```python
from build123d import *

# Parameters (mm, degrees)
ESBO_O1_W                = 35
ESBO_O1_H                = 20
RESSALTO_EXTRUS_O1_DEPTH = 5
ESBO_O2_W                = 5
ESBO_O2_H                = 20
RESSALTO_EXTRUS_O2_DEPTH = 30
ESBO_O4_W                = 42.3
ESBO_O4_H                = 5
RESSALTO_EXTRUS_O3_DEPTH = 50
ESBO_O5_W                = 7.3
ESBO_O5_H                = 5
RESSALTO_EXTRUS_O4_DEPTH = 35
ESBO_O6_R                = 3.1
ESBO_O6_R_2              = 12.5
CORTE_EXTRUS_O1_DEPTH    = 39
ESBO_O7_R                = 3
CORTE_EXTRUS_O2_DEPTH    = 36
ESBO_O8_R                = 3
CORTE_EXTRUS_O3_DEPTH    = 10


with BuildPart() as part:
    # Esboço1 → Ressalto-extrusão1 (new body)
    with BuildSketch(Plane.XY):
        with Locations((-76.705213928, -265)):
            Rectangle(ESBO_O1_W, ESBO_O1_H)
    extrude(amount=RESSALTO_EXTRUS_O1_DEPTH)

    # Esboço2 → Ressalto-extrusão2 (add)
    with BuildSketch(Plane(origin=(0, 0, 0), x_dir=(-1, 0, 0), z_dir=(0, 0, -1))):
        with Locations((61.705213928, -265)):
            Rectangle(ESBO_O2_W, ESBO_O2_H)
    extrude(amount=RESSALTO_EXTRUS_O2_DEPTH)

    # Esboço4 → Ressalto-extrusão3 (add)
    with BuildSketch(Plane(origin=(-59.205213928, 0, 0), x_dir=(0, 0, -1), z_dir=(1, 0, 0))):
        with Locations((8.85, -272.5)):
            Rectangle(ESBO_O4_W, ESBO_O4_H)
    extrude(amount=RESSALTO_EXTRUS_O3_DEPTH)

    # Esboço5 → Ressalto-extrusão4 (add)
    with BuildSketch(Plane.ZY.offset(59.205213928)):
        with Locations((8.65, -272.5)):
            Rectangle(ESBO_O5_W, ESBO_O5_H)
    extrude(amount=RESSALTO_EXTRUS_O4_DEPTH)

    # Esboço6 → Corte-extrusão1 (cut)
    with BuildSketch(Plane.XZ.offset(275)):
        with Locations((-14.555213928, 6.65)):
            Circle(ESBO_O6_R)
        with Locations((-45.555213928, -24.35)):
            Circle(ESBO_O6_R)
        with Locations((-30.055213928, -8.85)):
            Circle(ESBO_O6_R_2)
        with Locations((-45.555213928, 6.65)):
            Circle(ESBO_O6_R)
        with Locations((-14.555213928, -24.35)):
            Circle(ESBO_O6_R)
    extrude(amount=-CORTE_EXTRUS_O1_DEPTH, mode=Mode.SUBTRACT)

    # Esboço7 → Corte-extrusão2 (cut, through all)
    with BuildSketch(Plane(origin=(-59.205213928, 0, 0), x_dir=(0, 0, -1), z_dir=(1, 0, 0))):
        with Locations((21, -262.5)):
            Circle(ESBO_O7_R)
        with Locations((7, -262.5)):
            Circle(ESBO_O7_R)
    extrude(amount=-CORTE_EXTRUS_O2_DEPTH, mode=Mode.SUBTRACT)

    # Esboço8 → Corte-extrusão3 (cut)
    with BuildSketch(Plane.XY.offset(5)):
        with Locations((-71.205213928, -262.5)):
            Circle(ESBO_O8_R)
        with Locations((-86.205213928, -262.5)):
            Circle(ESBO_O8_R)
    extrude(amount=-CORTE_EXTRUS_O3_DEPTH, mode=Mode.SUBTRACT)


solid = part.part
```
Can you work these out from the model? Positions are in its coordinate system, mm. A direction names the side the tool comes from. Coordinates: 2 decimals unless noted, no trailing zeros. Loops run counter-clockwise (first coordinate to the right, second up) from the corner with the lowest first, then second, coordinate; pieces in that order, holes last. Notation, with made-up numbers: (43, 6) - (48, 6) arc R14 ccw to (48, 24) - close; hole circle Ø8 at (84, 70.5). An arc over 180 degrees is marked (long way). Use a Markdown table: item, result.
Item 1: I want a section at C-C on z = -2.5. Please give me the cut outline in (x, y).
Numbers:
| item | result |
|---|---|
| outline | (-64.21, -275) - (-40.82, -275) - (-40.82, -270) - (-59.21, -270) - (-59.21, -255) - (-64.21, -255) - close; (-19.29, -275) - (-9.21, -275) - (-9.21, -270) - (-19.29, -270) - close |
Item 2: I want a section at D-D on x = -85.5. Please give me the cut outline in (y, z), and give its area (3 significant figures).
Numbers:
| item | result |
|---|---|
| outline | (-275, 0) - (-265.42, 0) - (-265.42, 5) - (-270, 5) - (-270, 12.3) - (-275, 12.3) - close; (-259.58, 0) - (-255, 0) - (-255, 5) - (-259.58, 5) - close |
| area | 107 mm2 |
Item 3: I want a section at A-A on y = -262.5. Please give me the cut outline in (x, z).
Numbers:
| item | result |
|---|---|
| outline | (-94.21, 0) - (-89.21, 0) - (-89.21, 5) - (-94.21, 5) - close; (-83.21, 0) - (-74.21, 0) - (-74.21, 5) - (-83.21, 5) - close; (-68.21, 0) - (-64.21, 0) - (-64.21, -4) - (-59.21, -4) - (-59.21, 5) - (-68.21, 5) - close; (-64.21, -30) - (-59.21, -30) - (-59.21, -24) - (-64.21, -24) - close; (-64.21, -18) - (-59.21, -18) - (-59.21, -10) - (-64.21, -10) - close |
Item 4: I want a section at B-B on z = -8.85. Please give me the cut outline in (x, y), and give its area (3 significant figures).
Numbers:
| item | result |
|---|---|
| outline | (-64.21, -275) - (-42.56, -275) - (-42.56, -270) - (-59.21, -270) - (-59.21, -264.86) - (-64.21, -264.86) - close; (-64.21, -260.14) - (-59.21, -260.14) - (-59.21, -255) - (-64.21, -255) - close; (-17.56, -275) - (-9.21, -275) - (-9.21, -270) - (-17.56, -270) - close |
| area | 201 mm2 |
Item 5: For faces 5 (the face through (-18.13, -272.54, -5.1)), 6 (the face through (-79, -265, 0)), 7 (the face through (-61.67, -259.526, -20.609)), 8 (the face through (-59.205, -263, -12)), 9 (the face through (-77, -262, 5)), which set-ups out of +Z, -Z, +X, -X, +Y, -Y let a thin tool reach every point of the face, with its end or its side?
Numbers:
| item | result |
|---|---|
| face 5 | +Y, -Y |
| face 6 | -Z, -X, +Y, -Y |
| face 7 | +X, -X |
| face 8 | +Z, -Z, +X, +Y |
| face 9 | +Z, +X, -X, +Y |
Item 6: Will these pins go through, and if not, where does the flat tip stop? pin 1 (21 mm diameter, centred on x = -48, z = -17, fed in from +Y); pin 2 (5 mm diameter, centred on y = -260, z = -9.5, fed in from -X); pin 3 (5.5 mm diameter, centred on y = -262.5, z = -7, fed in from +X); pin 4 (9.5 mm diameter, centred on x = -71.21, y = -262.5, fed in from -Z).
Numbers:
| item | result |
|---|---|
| pin 1 | stops at y = -270 |
| pin 2 | stops at x = -64.21 |
| pin 3 | passes through |
| pin 4 | stops at z = 0 |
Item 7: If I drill on probe 1 along Z at (x, y) = (-62.2, -262.5); probe 2 along Y at (x, z) = (-61, -7); probe 3 along X at (y, z) = (-272.5, 7.5), over which ranges is the centre line in solid material (lowest first)? Write a range as from..to.
Numbers:
| item | result |
|---|---|
| probe 1 | z = -30..-24, -18..-10, -4..5 |
| probe 2 | y = -275..-265.5, -259.5..-255 |
| probe 3 | x = -94.21..-48.54, -42.57..-17.54, -11.57..-9.21 |
Item 8: We'd pull the mould along Y, two halves only. Please class faces 1 (the face through (-69, -255, 1)), 2 (the face through (-71.596, -259.526, 2.535)), 3 (the face through (-51, -275, -4)), 4 (the face through (-42.6, -272.54, 7.58)): released by +Y, released by -Y, zero draft, split by the parting line, or undercut.
Numbers:
| item | result |
|---|---|
| face 1 | released by +Y |
| face 2 | undercut |
| face 3 | released by -Y |
| face 4 | zero draft |
